Drawing for the job (mm, zero at the part's lowest x, y, z). A direction names the side the tool comes from. Give positions to 0.01 mm unless a question says otherwise; leave off trailing zeros. Loops run counter-clockwise (first coordinate to the right, second up) from the corner with the lowest first, then second, coordinate; pieces in that order, holes last. Notation, with made-up numbers: (22, -13.75) - (53, -13.75) arc R9 ccw to (53, -2.75) - close; hole circle Ø6 at (1, 31). An arc over 180 degrees is marked (long way). Return JSON: item names as keys, results as strings. Group by question number.
1) Slice it at B-B (y = 15). List the corners of the cut face in (x, z), and give its area (3 significant figures).
2) 3-axis set-ups, long thin cutter, end or side, ignore diameter. For the marked faces 1 and 2: which of +Z, -Z, +X, -X, +Y, -Y reach the whole face in a straight line?
3) Mould opens along Y. For the marked faces 3, 4 and 5 say: released by +Y, released by -Y, zero draft, split by the parting line, or undercut.
4) Slice it at A-A (x = 10). List the corners of the cut face in (y, z), and give its area (3 significant figures).
5) Drill centre lines: probe 1 along X at (y, z) = (24, 13); probe 2 along Y at (x, z) = (20.5, 36.5); probe 3 along Y at (x, z) = (27.5, 40.5). Where is each one in solid material? Low to high. Write a range as from..to.
6) Slice it at C-C (z = 36). List the corners of the cut face in (x, y), and give its area (3 significant figures).
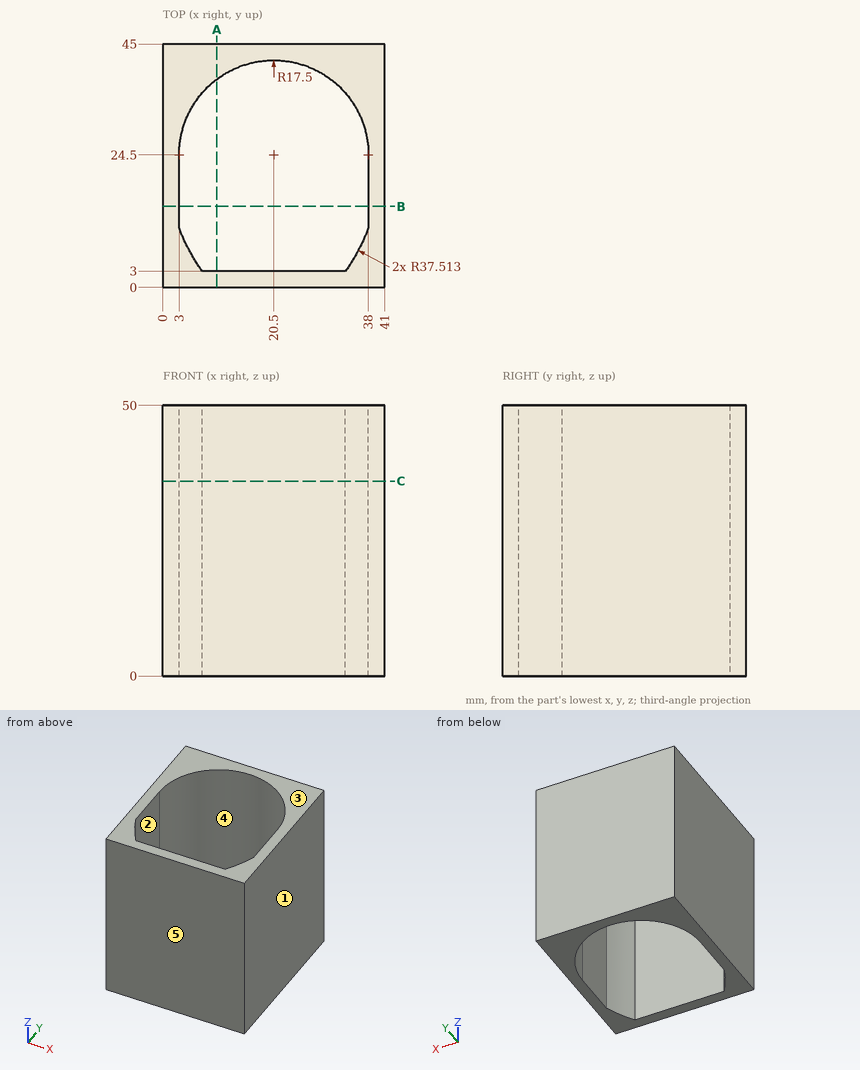
Results:
{
 "1": {"outline": "(0, 0) - (3, 0) - (3, 50) - (0, 50) - close; (38, 0) - (41, 0) - (41, 50) - (38, 50) - close", "area": "300 mm2"},
 "2": {"face 1": "+Z, -Z, +X, +Y, -Y", "face 2": "+Z, -Z"},
 "3": {"face 3": "zero draft", "face 4": "undercut", "face 5": "released by -Y"},
 "4": {"outline": "(0, 0) - (3, 0) - (3, 50) - (0, 50) - close; (38.5, 0) - (45, 0) - (45, 50) - (38.5, 50) - close", "area": "475 mm2"},
 "5": {"probe 1": "0..3, 38..41", "probe 2": "0..3, 42..45", "probe 3": "0..3, 40.54..45"},
 "6": {"outline": "(0, 0) - (41, 0) - (41, 45) - (0, 45) - close; hole (3, 11) arc R37.51 ccw to (7.26, 3) - (33.74, 3) arc R37.51 ccw to (38, 11) - (38, 24.5) arc R17.5 ccw to (3, 24.5) - close", "area": "642 mm2"}
}
